Read the model definition and answer for the solid it produces. Units are mm, in the model's axes. Face numbers are marked on the shaded views. A direction names the side the tool comes from. Give positions to 0.01 mm unless a question says otherwise; leave off trailing zeros. Write each loop counter-clockwise with the first axis right and the second up, starting at its lowest first coordinate (ties: lowest second). Pieces come first, ordered by that corner, then holes. Notation, with made-up numbers: (51.25, 39) - (76.25, 39) arc R26 cw to (76.25, 62) - close; hole circle Ø11 at (77.5, -15). An arc over 180 degrees is marked (long way). Answer as CSV lines item,"result".
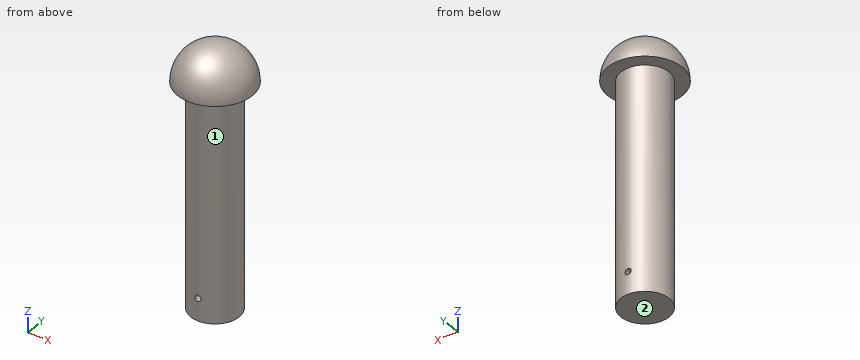
```python
from build123d import *

# Parameters (mm, degrees)
SKETCH1_R               = 9.75
BOSS_EXTRUDE1_DEPTH     = 90
REVOLVE1_ANGLE          = 180
CUT_EXTRUDE1_DEPTH      = 22
CUT_EXTRUDE1_DEPTH_BACK = 22
SKETCH3_R               = 1.221236648


with BuildPart() as part:
    # Sketch1 → Boss-Extrude1 (new body)
    with BuildSketch(Plane.XY):
        with Locations(Location((0, 0, 0), (0, 0, 180))):
            Circle(SKETCH1_R)
    extrude(amount=BOSS_EXTRUDE1_DEPTH)

    # Sketch2 → Revolve1 (revolve)
    with BuildSketch(Plane.XY.offset(90)):
        with BuildLine():
            Line((0, 15), (0, -15))
            ThreePointArc((0, -15), (15, 0), (0, 15))
        make_face()
    revolve(axis=Axis((0, 15, 90), (0, -1, 0)), revolution_arc=REVOLVE1_ANGLE)

    # Sketch3 → Cut-Extrude1 (cut, two sides: drawn at the far end of the back side and taken through both)
    with BuildSketch(Plane(origin=(0, 0, 0), x_dir=(1, 0, 0), z_dir=(0, 1, 0)).offset(-CUT_EXTRUDE1_DEPTH_BACK)):
        with Locations(Location((0.008150648, -9.023432345, 0), (0, 0, 90))):
            Circle(SKETCH3_R)
    extrude(amount=CUT_EXTRUDE1_DEPTH + CUT_EXTRUDE1_DEPTH_BACK, mode=Mode.SUBTRACT)


solid = part.part
```
(1) A cutting plane is placed at A-A (y = 0). Write down the section's boundary in (x, z).
Worked out:
outline,"(-15, 90) - (-9.75, 90) - (-9.75, 0) - (9.75, 0) - (9.75, 90) - (15, 90) arc R15 ccw to start; hole circle Ø2.44 at (0.01, 9.02)"
(2) A cutting plane is placed at B-B (z = 80). Write down the section's boundary in (x, y), and give its area (3 significant figures).
Worked out:
outline,"circle Ø19.5 at (0, 0)"
area,"299 mm^2"
(3) For the marked faces 1 and 2, determine the directions among +Z, -Z, +X, -X, +Y, -Y from which every point of the face is accessible in a straight line to the end or side of a thin tool.
Worked out:
face 1,"-Z"
face 2,"-Z, +X, -X, +Y, -Y"
(4) Find the intervals of material crossed by L1, parallel to Y at x = -0.25, z = 60; L2, parallel to Z at x = 9.5, y = -7.25, in increasing order.
Worked out:
L1,"y = -9.75 to 9.75"
L2,"z = 90 to 99.07"
(5) A cutting plane is placed at D-D (x = -10.75). Write down the section's boundary in (y, z).
Worked out:
outline,"(-10.46, 90) - (10.46, 90) arc R10.46 ccw to start"
(6) Each of these flat-tipped pins is pushed along its axis until it touches: P1, Ø1.5, axis at x = -9, z = 64.5, coming from the +Y side; P2, Ø8, axis at x = -11, z = 24.5, coming from the -Y side; P3, Ø6, axis at x = 12, z = 31, coming from the -Y side. Where does it stop, or does it pass through?
Worked out:
P1,"stops at y = 5.2"
P2,"stops at y = -6.79"
P3,"stops at y = -3.75"
(7) A cutting plane is placed at C-C (y = 11.5). Write down the section's boundary in (x, z), and give its area (3 significant figures).
Worked out:
outline,"(-9.63, 90) - (9.63, 90) arc R9.63 ccw to start"
area,"146 mm^2"
